CAD build for the part. Positions are in the model's coordinates, mm. Round coordinates to 2 decimals unless told otherwise and drop trailing zeros. Order: outer loops, then holes, each group sorted by start corner. A loop starts at its lowest first (then second) coordinate and runs counter-clockwise, first axis right, second up. Notation, with made-up numbers: (-25, -18.5) -> (24, -18.5) arc R22 ccw to (24, 18.5) -> close; hole circle Ø7 at (20, 82.25). An arc over 180 degrees is marked (long way). Return JSON: item names as keys, results as strings. Group by question number.
Q1. Flat gauge pin, fed straight in: pin 1 (1.6 mm diameter, centred on x = -15, y = 75, fed in from -Z). Where does the tip first touch, or does it go through?
Q2. Cut at C-C (z = 1.1). Count the separate pieces of the cut face and the enclosed holes in it, then the cut area to 3 significant figures.
Q3. Probe line 1 along Y through (x, z) = (0, 1.95); line 2 along X through (y, z) = (-5.5, 2.65); line 3 along Y through (x, z) = (11, 2.55). List the from-to ranges inside material, lowest first.
Q4. Cut at B-B (x = 38.5). Write the cut outline in (y, z).
Q5. Cut at A-A (y = 58). Write the cut outline in (x, z).
from build123d import *

# Parameters (mm, degrees)
F0_W     = 130
F0_H     = 170
F0_R     = 1.5
F1_DEPTH = 3


with BuildPart() as f1:
    # F0 (on Top) → F1 (new body)
    with BuildSketch(Plane.XY):
        Rectangle(F0_W, F0_H)
        with Locations((0, -80)):
            Circle(F0_R, mode=Mode.SUBTRACT)
        with BuildLine():
            ThreePointArc((-55, 74), (-55.707107, 75.707107), (-54, 75))
            Line((-54, 75), (-26, 75))
            ThreePointArc((-26, 75), (-25, 76), (-24, 75))
            ThreePointArc((-24, 75), (-24.292893, 74.292893), (-25, 74))
            Line((-25, 74), (-25, -74))
            ThreePointArc((-25, -74), (-24.292893, -74.292893), (-24, -75))
            ThreePointArc((-24, -75), (-25, -76), (-26, -75))
            Line((-26, -75), (-54, -75))
            ThreePointArc((-54, -75), (-55.707107, -75.707107), (-55, -74))
            Line((-55, -74), (-55, 74))
        make_face(mode=Mode.SUBTRACT)
        with BuildLine():
            ThreePointArc((-15, 74), (-15.707107, 75.707107), (-14, 75))
            Line((-14, 75), (14, 75))
            ThreePointArc((14, 75), (15, 76), (16, 75))
            ThreePointArc((16, 75), (15.707107, 74.292893), (15, 74))
            Line((15, 74), (15, -74))
            ThreePointArc((15, -74), (15.707107, -74.292893), (16, -75))
            ThreePointArc((16, -75), (15, -76), (14, -75))
            Line((14, -75), (-14, -75))
            ThreePointArc((-14, -75), (-15.707107, -75.707107), (-15, -74))
            Line((-15, -74), (-15, 74))
        make_face(mode=Mode.SUBTRACT)
        with BuildLine():
            ThreePointArc((25, 74), (24.292893, 75.707107), (26, 75))
            Line((26, 75), (54, 75))
            ThreePointArc((54, 75), (55, 76), (56, 75))
            ThreePointArc((56, 75), (55.707107, 74.292893), (55, 74))
            Line((55, 74), (55, -74))
            ThreePointArc((55, -74), (55.707107, -74.292893), (56, -75))
            ThreePointArc((56, -75), (55, -76), (54, -75))
            Line((54, -75), (26, -75))
            ThreePointArc((26, -75), (24.292893, -75.707107), (25, -74))
            Line((25, -74), (25, 74))
        make_face(mode=Mode.SUBTRACT)
        with Locations((0, 80)):
            Circle(F0_R, mode=Mode.SUBTRACT)
    extrude(amount=F1_DEPTH)


solid = f1.part
Solution:
{
 "1": {"pin 1": "passes through"},
 "2": {"separate pieces": "1", "enclosed holes": "5", "area": "8,560 mm²"},
 "3": {"line 1": "y = -85 to -81.5, -78.5 to -75, 75 to 78.5, 81.5 to 85", "line 2": "x = -65 to -55, -25 to -15, 15 to 25, 55 to 65", "line 3": "y = -85 to -75, 75 to 85"},
 "4": {"outline": "(-85, 0) -> (-75, 0) -> (-75, 3) -> (-85, 3) -> close; (75, 0) -> (85, 0) -> (85, 3) -> (75, 3) -> close"},
 "5": {"outline": "(-65, 0) -> (-55, 0) -> (-55, 3) -> (-65, 3) -> close; (-25, 0) -> (-15, 0) -> (-15, 3) -> (-25, 3) -> close; (15, 0) -> (25, 0) -> (25, 3) -> (15, 3) -> close; (55, 0) -> (65, 0) -> (65, 3) -> (55, 3) -> close"}
}
